Can you work these out from the model? Positions are in its coordinate system, mm. A direction names the side the tool comes from. Coordinates: 2 decimals unless noted, no trailing zeros. Order: outer loops, then holes, each group sorted by start corner. A loop starts at its lowest first (then second) coordinate and runs counter-clockwise, first axis right, second up. Notation, with made-up numbers: (-11, -35.5) - (44, -35.5) arc R21 cw to (44, -9.5) - close; hole circle Ø7 at (32, -20.5). An arc over 180 degrees is marked (long way). Return JSON: item names as keys, results as strings. Group by question number.
1) If I drill on line 1 along Z through (x, y) = (-13, 39); line 2 along Y through (x, z) = (-1.5, 14.5), over which ranges is the centre line in solid material (lowest first)?
2) Imagine slicing it at C-C (y = 46). Write out the boundary of the cut face in (x, z), and give its area (3 significant figures).
3) Which directions (+Z, -Z, +X, -X, +Y, -Y) give clear straight access to the entire face, cutting with the end or side of a thin tool? Please do faces 5 (the face through (13, 37.5, 13)), 6 (the face through (17.5, 20, 0)).
4) For pin 1 Ø0.9 at (x, z) = (-13, -13.5) entering from +Y; pin 2 Ø2.5 at (x, z) = (-13.5, 13.5) entering from +Y; pin 3 Ø1 at (x, z) = (4, -4.5) entering from +Y, each with a flat end and sliding along its axis, tell me the tip position at first contact or that it passes through.
5) Imagine slicing it at B-B (x = 0). Write out the boundary of the cut face in (y, z), and give its area (3 significant figures).
6) Imagine slicing it at D-D (z = 4). Write out the boundary of the cut face in (x, y), and give its area (3 significant figures).
7) Imagine slicing it at A-A (z = -13). Write out the boundary of the cut face in (x, y).
8) If we mould it in two halves opening along Z, with no side actions, what happens to faces 1 (the face through (13, 37.5, -13)), 2 (the face through (0, 20, -17.5)), 3 (the face through (0, 0, 0)), 4 (the face through (-13, 37.5, 13))? For each: pulls with the +Z half, pulls with the -Z half, needs draft (parallel to the pull), parting line crosses it, or undercut.
Autodesk Inventor part; units mm, degrees
ref_plane "YZ Plane" through (0, 0, 0) normal (1, 0, 0) x (0, 1, 0)
ref_plane "XZ Plane" through (0, 0, 0) normal (0, 1, 0) x (-1, 0, 0)
ref_plane "XY Plane" through (0, 0, 0) normal (0, 0, 1) x (1, 0, 0)
sketch "草圖1" plane through (0, 0, 0) normal (0, 1, 0) x (-1, 0, 0)
  line L0 (-17.5, 17.5) -> (17.5, 17.5)
  line L1 (17.5, 17.5) -> (17.5, -17.5)
  line L2 (17.5, -17.5) -> (-17.5, -17.5)
  line L3 (-17.5, -17.5) -> (-17.5, 17.5)
  line L4 (-17.5, 17.5) -> (17.5, -17.5) construction
  line L5 (17.5, 17.5) -> (-17.5, -17.5) construction
  point P0 (0, 0)
  dimension "d0" = 35
  dimension "d1" = 35
extrude "擠出1" add sketch "草圖1" along normal blind 40
sketch "草圖2" plane through (0, 40, 0) normal (0, 1, 0) x (1, 0, 0)
  circle A0 centre (0, 0) radius 11
  dimension "d4" = 22
extrude "擠出2" add sketch "草圖2" along normal blind 2
sketch "草圖3" plane through (0, 42, 0) normal (0, 1, 0) x (1, 0, 0)
  circle A0 centre (0, 0) radius 2.5
  dimension "d7" = 5
extrude "擠出3" add sketch "草圖3" along normal blind 18
sketch "草圖4" plane through (0, 40, 0) normal (0, 1, 0) x (1, 0, 0)
  line L0 (13, -13) -> (-13, -13) construction
  line L1 (-13, -13) -> (-13, 13) construction
  line L2 (-13, 13) -> (13, 13) construction
  line L3 (13, 13) -> (13, -13) construction
  line L4 (13, -13) -> (-13, 13) construction
  line L5 (-13, -13) -> (13, 13) construction
  circle A0 centre (-13, -13) radius 1.5
  circle A1 centre (13, -13) radius 1.5
  circle A2 centre (13, 13) radius 1.5
  circle A3 centre (-13, 13) radius 1.5
  point P0 (0, 0)
  dimension "d10" = 26
  dimension "d11" = 26
  dimension "d12" = 3
  dimension "d15" = 360
extrude "擠出4" cut sketch "草圖4" against normal blind 2.5
sketch "草圖5" plane through (0, 0, 0) normal (0, -1, 0) x (1, 0, 0)
  circle A0 centre (0, 0) radius 11
properties part number "35x40 stepper"
Calculated:
{
 "1": {"line 1": "-17.5 to -14.5, -11.5 to 11.5, 14.5 to 17.5", "line 2": "0 to 40"},
 "2": {"outline": "circle Ø5 at (0, 0)", "area": "19.6 mm2"},
 "3": {"face 5": "+Y", "face 6": "+Z, -Z, +X, +Y, -Y"},
 "4": {"pin 1": "y = 37.5", "pin 2": "y = 40", "pin 3": "y = 42"},
 "5": {"outline": "(0, -17.5) - (40, -17.5) - (40, -11) - (42, -11) - (42, -2.5) - (60, -2.5) - (60, 2.5) - (42, 2.5) - (42, 11) - (40, 11) - (40, 17.5) - (0, 17.5) - close", "area": "1,530 mm2"},
 "6": {"outline": "(-17.5, 0) - (17.5, 0) - (17.5, 40) - (10.25, 40) - (10.25, 42) - (-10.25, 42) - (-10.25, 40) - (-17.5, 40) - close", "area": "1,440 mm2"},
 "7": {"outline": "(-17.5, 0) - (17.5, 0) - (17.5, 40) - (14.5, 40) - (14.5, 37.5) - (11.5, 37.5) - (11.5, 40) - (-11.5, 40) - (-11.5, 37.5) - (-14.5, 37.5) - (-14.5, 40) - (-17.5, 40) - close"},
 "8": {"face 1": "undercut", "face 2": "pulls with the -Z half", "face 3": "needs draft", "face 4": "undercut"}
}
